Design review of the part built by this model. Coordinates are the model's own, in mm. Face numbers are marked on the shaded views. Round coordinates to 2 decimals unless told otherwise and drop trailing zeros. Loops run counter-clockwise (first coordinate to the right, second up) from the corner with the lowest first, then second, coordinate; pieces in that order, holes last. Notation, with made-up numbers: M 68.5,38.5 L 115.5,38.5 A21 ccw 115.5,74.5 Z; hole C 85.5,25 d9. An arc over 180 degrees is marked long. Use a Markdown table: item, result.
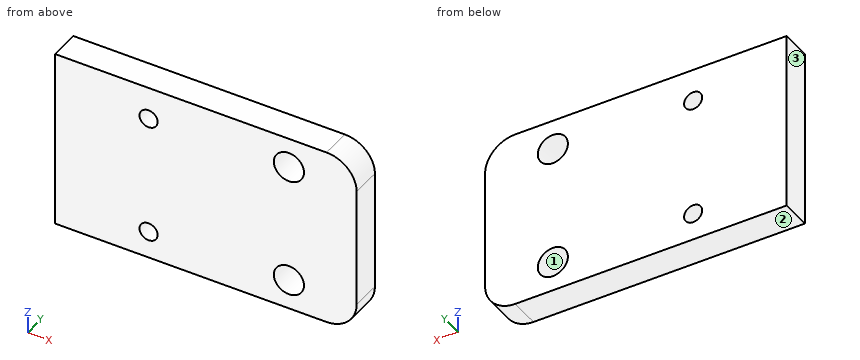
from build123d import *

# Parameters (mm, degrees)
SKETCH1_W           = 50
SKETCH1_H           = 30
SKETCH1_R           = 1.5
BOSS_EXTRUDE1_DEPTH = 5
FILLET1_R           = 5
SKETCH2_R           = 2.5
CUT_EXTRUDE1_DEPTH  = 9


with BuildPart() as part:
    # Sketch1 → Boss-Extrude1 (new body)
    with BuildSketch(Plane(origin=(0, 0, 0), x_dir=(1, 0, 0), z_dir=(0, 1, 0))):
        with Locations((-25, 15)):
            Rectangle(SKETCH1_W, SKETCH1_H)
        with Locations(Location((-34.5, 5.45, 0), (0, 0, 270))):
            Circle(SKETCH1_R, mode=Mode.SUBTRACT)
        with Locations(Location((-34.5, 25.45, 0), (0, 0, 270))):
            Circle(SKETCH1_R, mode=Mode.SUBTRACT)
    extrude(amount=BOSS_EXTRUDE1_DEPTH)

    # Fillet1
    fillet1_edges = [part.edges().sort_by_distance(p)[0] for p in [
        (0, 2.5, 0),
        (0, 2.5, -30),
    ]]
    fillet(fillet1_edges, radius=FILLET1_R)

    # Sketch2 → Cut-Extrude1 (cut)
    with BuildSketch(Plane.XZ):
        with Locations(Location((-11.23257698, -5, 0), (0, 0, 270))):
            Circle(SKETCH2_R)
        with Locations(Location((-11.23257698, -25, 0), (0, 0, 270))):
            Circle(SKETCH2_R)
    extrude(amount=-CUT_EXTRUDE1_DEPTH, mode=Mode.SUBTRACT)


solid = part.part
1. Take a section at A-A on z = -5.5. Give the boundary of the cut face in (x, y), and give its area (3 significant figures).
Check values:
| item | result |
|---|---|
| outline | M -50,0 L -36,0 L -36,5 L -50,5 Z; M -33,0 L -13.68,0 L -13.68,5 L -33,5 Z; M -8.78,0 L 0,0 L 0,5 L -8.78,5 Z |
| area | 211 mm² |
2. Insertion check: pin 1 (8 mm diameter, centred on x = -44.5, z = -24, fed in from -Y). The pin has a flat end and moves straight along its axis. Give the tip position at first contact, or say it passes through.
Check values:
| item | result |
|---|---|
| pin 1 | stops at y = 0 |
3. Take a section at C-C on z = -24.5. Give the boundary of the cut face in (x, y).
Check values:
| item | result |
|---|---|
| outline | M -50,0 L -35.66,0 L -35.66,5 L -50,5 Z; M -33.34,0 L -13.68,0 L -13.68,5 L -33.34,5 Z; M -8.78,0 L 0,0 L 0,5 L -8.78,5 Z |
4. The part is to be moulded in two halves that separate along Z. For the marked faces 1, 2 and 3, say which applies: pulls with the +Z half, pulls with the -Z half, needs draft (parallel to the pull), parting line crosses it, or undercut.
Check values:
| item | result |
|---|---|
| face 1 | undercut |
| face 2 | pulls with the -Z half |
| face 3 | needs draft |
5. Take a section at B-B on y = 4.4. Give the boundary of the cut face in (x, z), and give its area (3 significant figures).
Check values:
| item | result |
|---|---|
| outline | M -50,-30 L -5,-30 A5 ccw 0,-25 L 0,-5 A5 ccw -5,0 L -50,0 Z; hole C -34.5,-25.45 d3; hole C -34.5,-5.45 d3; hole C -11.23,-25 d5; hole C -11.23,-5 d5 |
| area | 1,440 mm² |
6. Wall thickness on line 1 along Z through (x, y) = (-11, 0.8); line 2 along X through (y, z) = (3.95, -5.45); line 3 along Z through (x, y) = (-13, 2): over which ranges is each line inside the solid? List them lowest first. Write a range as from..to.
Check values:
| item | result |
|---|---|
| line 1 | z = -30..-27.49, -22.51..-7.49, -2.51..0 |
| line 2 | x = -50..-36, -33..-13.69, -8.77..0 |
| line 3 | z = -30..-26.77, -23.23..-6.77, -3.23..0 |
